```python
from build123d import *

# Parameters (mm, degrees)
RESSALTO_EXTRUS_O1_DEPTH = 2
ESBO_O2_R                = 1.5
ESBO_O2_R_2              = 1
ESBO_O2_W                = 14
ESBO_O2_H                = 1.527880785
CORTE_EXTRUS_O1_DEPTH    = 3.0000001


with BuildPart() as part:
    # Esboço1 → Ressalto-extrusão1 (new body)
    with BuildSketch(Plane(origin=(0, 0, 0), x_dir=(0, 0, -1), z_dir=(1, 0, 0))):
        with BuildLine():
            Line((-13, 34), (0, 34))
            Line((0, 34), (0, -15))
            ThreePointArc((0, -15), (-12.895532653, -7.661934325), (-13.173963237, 7.172634986))
            add(Edge.make_bspline(
                [(-13, 27), (-9.354199414, 16.239964162), (-13.173963237, 7.172634986)],
                knots=[0, 0, 0, 0.912495845, 0.912495845, 0.912495845], degree=2))
            Line((-13, 27), (-13, 34))
        make_face()
    ressalto_extrus_o1 = extrude(amount=RESSALTO_EXTRUS_O1_DEPTH)

    # Espelhar1: Ressalto-extrusão1 across plane
    add(ressalto_extrus_o1.mirror(Plane(origin=(2, 34, 0), x_dir=(1, 0, 0), z_dir=(0, 0, 1))))

    # Esboço2 → Corte-extrusão1 (cut, through all)
    with BuildSketch(Plane(origin=(2, 0, 0), x_dir=(0, 0, -1), z_dir=(1, 0, 0))):
        Circle(ESBO_O2_R)
        with Locations((11, 0)):
            Circle(ESBO_O2_R_2)
        with Locations((-11, 0)):
            Circle(ESBO_O2_R_2)
        with Locations((0, 30.236059608)):
            Rectangle(ESBO_O2_W, ESBO_O2_H)
        with BuildLine():
            Line((-9.810708435, 5), (-9.219544457, 5))
            ThreePointArc((-9.219544457, 5), (-8.742813163, 5.120950927), (-8.381404052, 5.454545455))
            ThreePointArc((-8.381404052, 5.454545455), (0, 10), (8.381404052, 5.454545455))
            ThreePointArc((8.381404052, 5.454545455), (8.742813163, 5.120950927), (9.219544457, 5))
            Line((9.219544457, 5), (9.810708435, 5))
            ThreePointArc((9.810708435, 5), (10.682986811, 5.510990353), (10.663813516, 6.52173913))
            ThreePointArc((10.663813516, 6.52173913), (0, 12.5), (-10.663813516, 6.52173913))
            ThreePointArc((-10.663813516, 6.52173913), (-10.682986811, 5.510990353), (-9.810708435, 5))
        make_face()
        with BuildLine():
            Line((-9.996736389, -4.616845413), (-9.40601466, -4.639707772))
            ThreePointArc((-9.40601466, -4.639707772), (-8.934317599, -4.779005068), (-8.586080114, -5.126326976))
            ThreePointArc((-8.586080114, -5.126326976), (-0.386734657, -9.992519017), (8.164187762, -5.77460286))
            ThreePointArc((8.164187762, -5.77460286), (8.538227759, -5.455234837), (9.019280003, -5.352811245))
            Line((9.019280003, -5.352811245), (9.610001733, -5.375673604))
            ThreePointArc((9.610001733, -5.375673604), (10.461865791, -5.920015714), (10.403617681, -6.929266854))
            ThreePointArc((10.403617681, -6.929266854), (-0.483418321, -12.490648771), (-10.90805419, -6.104453603))
            ThreePointArc((-10.90805419, -6.104453603), (-10.888123983, -5.093719467), (-9.996736389, -4.616845413))
        make_face()
    extrude(amount=-CORTE_EXTRUS_O1_DEPTH, mode=Mode.SUBTRACT)


solid = part.part
```
Geometry check sheet. Reference: the model listing, model coordinates, mm. A direction names the side the tool comes from. Round coordinates to 2 decimals unless told otherwise and drop trailing zeros. Order: outer loops, then holes, each group sorted by start corner. A loop starts at its lowest first (then second) coordinate and runs counter-clockwise, first axis right, second up. Notation, with made-up numbers: (-13.5, -9) -> (-4.5, -9) arc R15 cw to (-4.5, 19) -> close; hole circle Ø8 at (-17.75, 86.5). An arc over 180 degrees is marked (long way). Return JSON: item names as keys, results as strings. Group by question number.
Q1. Section check C-C, the plane x = 1.65. Count the separate pieces of the cut face and the enclosed holes in it, plus the area to 3 significant figures.
Q2. Release check for a two-part mould opening along Z. For faces 4 (the flat face through (1, 30, -13)), 5 (the flat face through (0, 9.8, 0.2)), 6 (the cylindrical face through (1, 10, 0)) record: released by +Z, released by -Z, zero draft, split by the parting line, or undercut.
Q3. Section check A-A, the plane y = 0. Record the boundary of the cut face in (x, z).
Q4. Section check D-D, the plane y = -8. Record the boundary of the cut face in (x, z).
Q5. Section check B-B, the plane z = -7.5. Record the boundary of the cut face in (x, y).
Q6. Tool access check on faces 1 (the flat face through (1, 30, 13)), 2 (the flat face through (2, 9.8, 0.2)), 3 (the cylindrical face through (1.01, 5.52, 10.69)). Record the directions out of +Z, -Z, +X, -X, +Y, -Y that give a thin tool (end or side, any length) a straight path to the whole face; none if there is none.
Q7. Gauge pin test, flat ends, axial feed: pin 1 (0.8 mm diameter, centred on x = 1.5, y = 30.5, fed in from +Z); pin 2 (1.2 mm diameter, centred on x = 1, y = 30.5, fed in from -Z); pin 3 (1.8 mm diameter, centred on y = 0, z = 0, fed in from -X); pin 4 (4 mm diameter, centred on y = -2.5, z = 11, fed in from -X). Record the tip position at first contact, or that the pin passes through.
Q8. Material ranges on probe 1 along Y at (x, z) = (1.65, 0); probe 2 along Y at (x, z) = (0.55, -8.5); probe 3 along Y at (x, z) = (1.4, 7.5), recorded low to high. Write a range as from..to.
Numbers:
{
 "1": {"separate pieces": "1", "enclosed holes": "6", "area": "1,050 mm^2"},
 "2": {"face 4": "released by -Z", "face 5": "zero draft", "face 6": "undercut"},
 "3": {"outline": "(0, -15) -> (2, -15) -> (2, -12) -> (0, -12) -> close; (0, -10) -> (2, -10) -> (2, -1.5) -> (0, -1.5) -> close; (0, 1.5) -> (2, 1.5) -> (2, 10) -> (0, 10) -> close; (0, 12) -> (2, 12) -> (2, 15) -> (0, 15) -> close"},
 "4": {"outline": "(0, -12.69) -> (2, -12.69) -> (2, -9.6) -> (0, -9.6) -> close; (0, -6) -> (2, -6) -> (2, 6) -> (0, 6) -> close; (0, 9.6) -> (2, 9.6) -> (2, 12.69) -> (0, 12.69) -> close"},
 "5": {"outline": "(0, -12.99) -> (2, -12.99) -> (2, -10) -> (0, -10) -> close; (0, -6.61) -> (2, -6.61) -> (2, 6.61) -> (0, 6.61) -> close; (0, 10) -> (2, 10) -> (2, 34) -> (0, 34) -> close"},
 "6": {"face 1": "+Z, +X, -X, +Y", "face 2": "+Z, -Z, +X, +Y, -Y", "face 3": "+X, -X"},
 "7": {"pin 1": "z = 13", "pin 2": "z = -13", "pin 3": "through", "pin 4": "x = 0"},
 "8": {"probe 1": "-15..-12.5, -10..-1.5, 1.5..10, 12.5..29.47, 31..34", "probe 2": "-12.36..-9.17, -5.48..5.31, 9.17..34", "probe 3": "-12.99..-10, -6.61..6.61, 10..34"}
}
